Design review of the part shown in the three views and the two pictorial views. Dimensions are in mm from the part's minimum x, y and z. A direction names the side the tool comes from. Round coordinates to 2 decimals unless told otherwise and drop trailing zeros. Loops run counter-clockwise (first coordinate to the right, second up) from the corner with the lowest first, then second, coordinate; pieces in that order, holes last. Notation, with made-up numbers: (-18.5, -25) -> (26.5, -25) arc R25 ccw to (26.5, -6) -> close; hole circle Ø3 at (40.25, -7). An arc over 180 degrees is marked (long way). Write each question's results on one line, items separated by ' | '. Start each with the question number.
Item 1: Clearance check with flat-ended pins moving along their axes: pin 1 Ø3 at (x, y) = (18.5, 4) entering from +Z; pin 2 Ø0.9 at (y, z) = (0.5, 4.5) entering from +X; pin 3 Ø1.5 at (x, z) = (22.5, 7.5) entering from -Y. State where each tip first meets the part, or that it passes through.
Item 2: We need section C-C (x = 23.5). Give the boundary of the cut face in (y, z).
Item 3: We need section A-A (z = 4.85). Give the boundary of the cut face in (x, y), and give its area (3 significant figures).
Item 4: Tool access review of the marked faces 1 and 2: name each direction out of +Z, -Z, +X, -X, +Y, -Y from which nothing blocks a thin tool from reaching the whole face with its end or side.
Item 5: We need section B-B (y = 6.5). Give the boundary of the cut face in (x, z), and give its area (3 significant figures).
Item 6: We need section D-D (z = 3.5). Give the boundary of the cut face in (x, y), and give its area (3 significant figures).
Item 7: For L1, parallel to X at y = 9.75, z = 2.25; L2, parallel to X at y = 0.75, z = 4.75; L3, parallel to Z at x = 26.5, y = 4.25, list the stretches that pass through material, from the lowest coordinate up. Write a range as from..to.
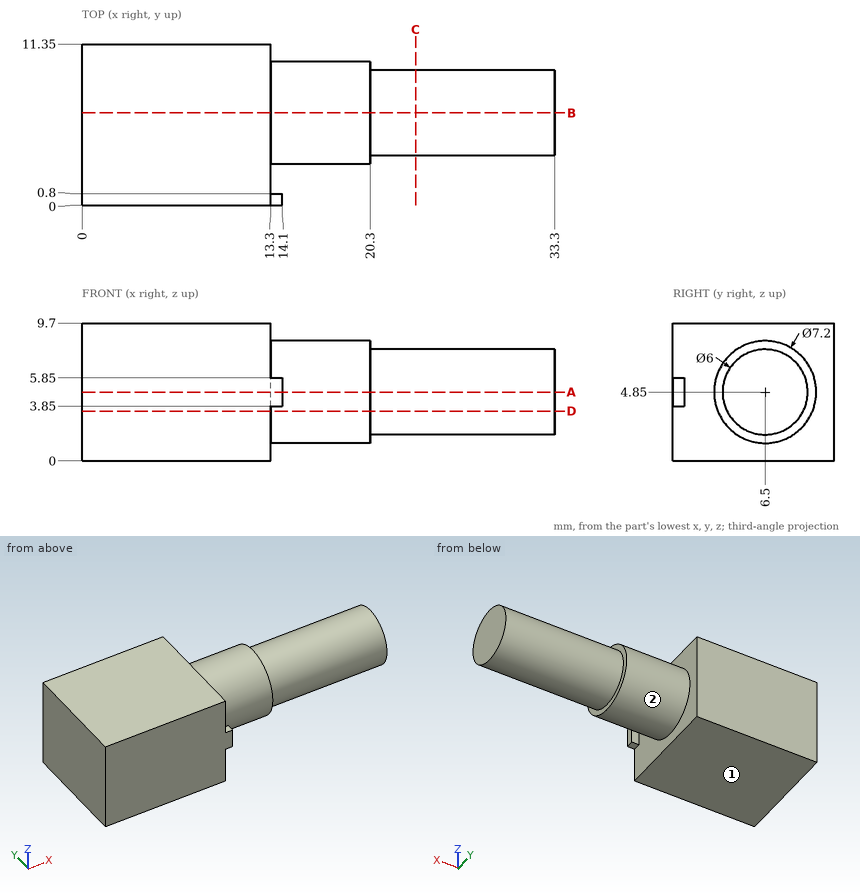
Here are the results:
1) pin 1: stops at z = 8.31 | pin 2: stops at x = 14.1 | pin 3: stops at y = 4.18
2) outline: circle Ø6 at (6.5, 4.85)
3) outline: (0, 0) -> (14.1, 0) -> (14.1, 0.8) -> (13.3, 0.8) -> (13.3, 2.9) -> (20.3, 2.9) -> (20.3, 3.5) -> (33.3, 3.5) -> (33.3, 9.5) -> (20.3, 9.5) -> (20.3, 10.1) -> (13.3, 10.1) -> (13.3, 11.35) -> (0, 11.35) -> close | area: 280 mm2
4) face 1: -Z, +X, -X, +Y, -Y | face 2: +X
5) outline: (0, 0) -> (13.3, 0) -> (13.3, 1.25) -> (20.3, 1.25) -> (20.3, 1.85) -> (33.3, 1.85) -> (33.3, 7.85) -> (20.3, 7.85) -> (20.3, 8.45) -> (13.3, 8.45) -> (13.3, 9.7) -> (0, 9.7) -> close | area: 257 mm2
6) outline: (0, 0) -> (13.3, 0) -> (13.3, 3.16) -> (20.3, 3.16) -> (20.3, 3.82) -> (33.3, 3.82) -> (33.3, 9.18) -> (20.3, 9.18) -> (20.3, 9.84) -> (13.3, 9.84) -> (13.3, 11.35) -> (0, 11.35) -> close | area: 267 mm2
7) L1: x = 0..13.3 | L2: x = 0..14.1 | L3: z = 2.87..6.83
